Source: CAD feature listing. Evaluate the final solid. Frame: model axes, mm. A direction names the side the tool comes from. Give positions to 0.01 mm unless a question says otherwise; leave off trailing zeros. Order: outer loops, then holes, each group sorted by start corner. A loop starts at its lowest first (then second) coordinate and runs counter-clockwise, first axis right, second up. Notation, with made-up numbers: M 62.5,48.25 L 74.5,48.25 A6 ccw 74.5,59.25 Z; hole C 85.25,27 d10. An arc over 180 degrees is marked long. Answer in a Markdown table with one row per item. Add a question column.
(1) Section query C-C, the plane z = 2.8. Return loops of the section in (x, y) (3 decimals), plus the area to 3 significant figures.
(2) Section query D-D, the plane x = 14.5. Return loops of the section in (y, z), plus the area to 3 significant figures.
(3) Section query A-A, the plane x = 10.5. Return loops of the section in (y, z) (3 decimals), plus the area to 3 significant figures.
(4) Section query B-B, the plane z = 5.75. Return loops of the section in (x, y) (3 decimals).
(5) Mould query, pull axis Z, two halves, no side actions, for faces 1 (the face through (9.53, 33.74, 3.55)), 2 (the face through (21, 15, 6)), 3 (the face through (33.226, 12.769, 3.938)), 4 (the face through (20, 13, 0)). Classes: pulls with the +Z half, pulls with the -Z half, needs draft (parallel to the pull), parting line crosses it, or undercut.
(6) Material intervals for line 1 along X through (y, z) = (32.5, 2.75) (3 decimals); line 2 along Y through (x, z) = (19.75, 4.5); line 3 along Y through (x, z) = (14.5, 10.25), sorted ascending.
(7) Pin query (flat end, axial travel): P1, Ø12, axis at x = 26.5, y = 16.5, coming from the -Z side; P2, Ø1.5, axis at y = 28, z = 12, coming from the -X side; P3, Ø5, axis at x = 28, y = 25.5, coming from the -Z side; P4, Ø6, axis at y = 20, z = 12.5, coming from the +X side (3 decimals). Return the tip coordinate at first contact, or that it passes through.
(8) Set-up query: faces 5 (the face through (20, 23, 7.5)), 6 (the face through (10, 20, 11)), 7 (the face through (11.226, 12.769, 3.938)), 8 (the face through (21, 31, 6)), 9 (the face through (6.525, 13, 7)). Return all of +Z, -Z, +X, -X, +Y, -Y with unobstructed straight access to the full face (end or side cutting, diameter ignored); none if empty.
Autodesk Inventor part; units mm, degrees
ref_plane "YZ Plane" through (0, 0, 0) normal (1, 0, 0) x (0, 1, 0)
ref_plane "XZ Plane" through (0, 0, 0) normal (0, 1, 0) x (-1, 0, 0)
ref_plane "XY Plane" through (0, 0, 0) normal (0, 0, 1) x (1, 0, 0)
sketch "스케치1" plane through (0, 0, 0) normal (0, 0, 1) x (1, 0, 0)
  line L0 (7.5, 38) -> (7.5, 36.5)
  line L1 (2, 38) -> (7.5, 38)
  line L2 (2, 38) -> (2, 8)
  line L3 (2, 8) -> (6.525, 8)
  line L4 (6.525, 10.5) -> (6.525, 8)
  line L5 (6.525, 10.5) -> (10.3997, 10.5)
  line L6 (10.3997, 10.5) -> (10.6003, 10.5)
  line L7 (10.6003, 10.5) -> (14.475, 10.5)
  line L8 (14.475, 10.5) -> (14.475, 8)
  line L9 (14.475, 8) -> (28.525, 8)
  line L10 (28.525, 10.5) -> (28.525, 8)
  line L11 (28.525, 10.5) -> (32.3997, 10.5)
  line L12 (32.3997, 10.5) -> (32.6003, 10.5)
  line L13 (32.6003, 10.5) -> (34.7876, 10.5)
  line L14 (34.7876, 10.5) -> (34.7876, 19.4)
  line L15 (36, 19.4) -> (34.7876, 19.4)
  line L16 (36, 24) -> (36, 19.4)
  line L17 (38.55, 24) -> (36, 24)
  line L18 (38.55, 24) -> (38.55, 25.4)
  line L19 (38.55, 25.4) -> (37.1, 25.4)
  line L20 (37.1, 25.4) -> (37.1, 35.5)
  line L21 (49.9, 35.5) -> (37.1, 35.5)
  line L22 (49.9, 25.4) -> (49.9, 35.5)
  line L23 (49.9, 25.4) -> (48.45, 25.4)
  line L24 (48.45, 24) -> (48.45, 25.4)
  line L25 (51, 24) -> (48.45, 24)
  line L26 (51, 24) -> (51, 10.5)
  line L27 (51, 10.5) -> (54.3997, 10.5)
  line L28 (54.3997, 10.5) -> (54.6003, 10.5)
  line L29 (54.6003, 10.5) -> (57.5, 10.5)
  line L30 (57.5, 36.5) -> (57.5, 10.5)
  line L31 (57.5, 36.5) -> (51.5, 36.5)
  line L32 (51.5, 38) -> (51.5, 36.5)
  line L33 (35.5, 38) -> (51.5, 38)
  line L34 (35.5, 36.5) -> (35.5, 38)
  line L35 (35.5, 36.5) -> (29.5, 36.5)
  line L36 (29.5, 38) -> (29.5, 36.5)
  line L37 (13.5, 38) -> (29.5, 38)
  line L38 (13.5, 36.5) -> (13.5, 38)
  line L39 (13.5, 36.5) -> (7.5, 36.5)
  line L40 (22.05, 14.2) -> (27.95, 14.2)
  line L41 (22.05, 18) -> (22.05, 14.2)
  line L42 (27.95, 18) -> (22.05, 18)
  line L43 (27.95, 14.2) -> (27.95, 18)
  line L44 (34.6876, 10.6) -> (7.6, 10.6)
  line L45 (7.6, 10.6) -> (7.6, 36.4)
  line L46 (7.6, 36.4) -> (34.6876, 36.4)
  line L47 (34.6876, 36.4) -> (34.6876, 10.6)
  line L48 (7.6, 36.4) -> (6.525, 36.4)
  line L49 (7.6, 10.6) -> (6.525, 10.6)
  line L50 (6.525, 10.6) -> (6.525, 36.4)
  line L51 (6.525, 36.4) -> (7.6, 36.4)
  line L52 (7.6, 36.4) -> (7.6, 10.6)
  point P0 (0, 0)
extrude "돌출1" add sketch "스케치1" along normal blind 15 contours L41 L42 L43 L40 | L44 L45 L46 L47 | L49 L50 L48 L45
sketch "스케치2" plane through (0, 0, 15) normal (0, 0, 1) x (1, 0, 0)
  line L0 (34.5, 38) -> (52.5, 38)
  line L1 (52.5, 38) -> (52.5, 36.5)
  line L2 (56.5, 36.5) -> (52.5, 36.5)
  line L3 (56.5, 38) -> (56.5, 36.5)
  line L4 (56.5, 38) -> (59.1, 38)
  line L5 (59.1, 38) -> (59.1, 40)
  line L6 (6, 40) -> (59.1, 40)
  line L7 (6, 38) -> (6, 40)
  line L8 (6, 38) -> (8.5, 38)
  line L9 (8.5, 38) -> (8.5, 36.5)
  line L10 (12.5, 36.5) -> (8.5, 36.5)
  line L11 (12.5, 38) -> (12.5, 36.5)
  line L12 (12.5, 38) -> (30.5, 38)
  line L13 (30.5, 38) -> (30.5, 36.5)
  line L14 (34.5, 36.5) -> (30.5, 36.5)
  line L15 (34.5, 38) -> (34.5, 36.5)
  line L16 (14.475, 10.5) -> (12.975, 10.5)
  line L17 (12.975, 10.5) -> (12.975, 8.5)
  line L18 (12.975, 8.5) -> (8.025, 8.5)
  line L19 (8.025, 10.5) -> (8.025, 8.5)
  line L20 (8.025, 10.5) -> (6.525, 10.5)
  line L21 (6.525, 10.5) -> (6.525, 8)
  line L22 (6, 8) -> (6.525, 8)
  line L23 (6, 8) -> (6, 6)
  line L24 (6, 6) -> (59.1, 6)
  line L25 (59.1, 8) -> (59.1, 6)
  line L26 (58.475, 8) -> (59.1, 8)
  line L27 (58.475, 8) -> (58.475, 10.5)
  line L28 (58.475, 10.5) -> (56.975, 10.5)
  line L29 (56.975, 10.5) -> (56.975, 8.5)
  line L30 (56.975, 8.5) -> (52.025, 8.5)
  line L31 (52.025, 10.5) -> (52.025, 8.5)
  line L32 (52.025, 10.5) -> (50.525, 10.5)
  line L33 (50.525, 10.5) -> (50.525, 8)
  line L34 (36.475, 8) -> (50.525, 8)
  line L35 (36.475, 8) -> (36.475, 10.5)
  line L36 (36.475, 10.5) -> (34.975, 10.5)
  line L37 (34.975, 10.5) -> (34.975, 8.5)
  line L38 (34.975, 8.5) -> (30.025, 8.5)
  line L39 (30.025, 10.5) -> (30.025, 8.5)
  line L40 (30.025, 10.5) -> (28.525, 10.5)
  line L41 (28.525, 10.5) -> (28.525, 8)
  line L42 (14.475, 8) -> (28.525, 8)
  line L43 (14.475, 8) -> (14.475, 10.5)
  line L44 (14.475, 36.4) -> (28.525, 36.4)
  line L45 (34.6876, 10.6) -> (34.6876, 36.4)
  line L46 (14.475, 10.6) -> (28.525, 10.6)
  line L47 (28.525, 10.6) -> (28.525, 36.4)
  line L48 (28.525, 36.4) -> (14.475, 36.4)
  line L49 (-13.0231, 23) -> (78.1205, 23)
  line L50 (14.5, -11.1) -> (14.5, 56.1)
  line L51 (34.6876, 36.4) -> (6.525, 36.4)
  line L52 (6.525, 36.4) -> (6.525, 10.6)
  line L53 (6.525, 10.6) -> (34.6876, 10.6)
  line L54 (28.525, 23) -> (34.6876, 23)
  line L55 (34.6876, 23) -> (34.6876, 31)
  line L56 (34.6876, 31) -> (28.525, 31)
  line L57 (28.525, 31) -> (28.525, 23)
  line L58 (28.525, 23) -> (34.6876, 23)
  line L59 (34.6876, 23) -> (34.6876, 15)
  line L60 (34.6876, 15) -> (28.525, 15)
  line L61 (28.525, 15) -> (28.525, 23)
  line L62 (6.525, 23) -> (12.688, 23)
  line L63 (12.688, 23) -> (12.688, 31)
  line L64 (12.688, 31) -> (6.525, 31)
  line L65 (6.525, 31) -> (6.525, 23)
  line L66 (14.5, 57.1) -> (14.5, -10.1)
  line L67 (12.688, 23) -> (12.688, 15)
  line L68 (12.688, 15) -> (6.525, 15)
  line L69 (6.525, 15) -> (6.525, 23)
  line L70 (6.525, 36.4) -> (6.525, 10.6)
  line L71 (12.688, 23) -> (6.525, 23)
  line L72 (6.525, 23) -> (6.525, 26)
  line L73 (6.525, 26) -> (12.688, 26)
  line L74 (12.688, 26) -> (12.688, 23)
  line L75 (12.688, 23) -> (6.525, 23)
  line L76 (6.525, 23) -> (6.525, 20)
  line L77 (6.525, 20) -> (12.688, 20)
  line L78 (12.688, 20) -> (12.688, 23)
  point P0 (0, 0)
  dimension "d3" = 6.163
  dimension "d4" = 8
extrude "돌출2" cut sketch "스케치2" against normal up to next contours L56 L45 L49 L47 | L49 L45 L60 L47 | L64 L63 L73 L52 | L67 L68 L52 L77
sketch "스케치4" plane through (6.525, 10.6, 0) normal (0, -1, 0) x (1, 0, 0)
  circle A0 centre (3.975, 2.8) radius 1.35
  circle A1 centre (25.975, 2.8) radius 1.35
  circle A2 centre (25.975, 2.8) radius 1.55
  circle A3 centre (3.975, 2.8) radius 1.55
  point P0 (-6.525, 0)
  dimension "d14" = 0.2
  dimension "d15" = 0.2
extrude "돌출4" cut sketch "스케치4" against normal up to next contours A0 | A1
sketch "스케치5" plane through (6.525, 36.4, 0) normal (0, 1, 0) x (1, 0, 0)
  circle A0 centre (25.975, -2.8) radius 1.025
  circle A1 centre (3.975, -2.8) radius 1.025
  circle A2 centre (25.975, -2.8) radius 1.225
  circle A3 centre (3.975, -2.8) radius 1.225
  point P0 (-6.525, 0)
  dimension "d16" = 0.2
  dimension "d17" = 0.2
extrude "돌출5" cut sketch "스케치5" against normal up to next contours A0 | A1 | A2 | A3
sketch "스케치6" plane through (0, 0, 0) normal (0, 0, -1) x (-1, 0, 0)
  line L0 (-28.525, 31) -> (-34.6876, 31)
  line L1 (-34.6876, 31) -> (-34.6876, 36.4)
  line L2 (-34.6876, 36.4) -> (-6.525, 36.4)
  line L3 (-6.525, 36.4) -> (-6.525, 31)
  line L4 (-6.525, 31) -> (-12.688, 31)
  line L5 (-12.688, 31) -> (-12.688, 26)
  line L6 (-12.688, 26) -> (-6.525, 26)
  line L7 (-6.525, 26) -> (-6.525, 20)
  line L8 (-6.525, 20) -> (-12.688, 20)
  line L9 (-12.688, 20) -> (-12.688, 15)
  line L10 (-12.688, 15) -> (-6.525, 15)
  line L11 (-6.525, 15) -> (-6.525, 10.6)
  line L12 (-6.525, 10.6) -> (-34.6876, 10.6)
  line L13 (-34.6876, 10.6) -> (-34.6876, 15)
  line L14 (-34.6876, 15) -> (-28.525, 15)
  line L15 (-28.525, 15) -> (-28.525, 31)
  line L16 (-12.688, 31) -> (-28.525, 31)
  line L17 (-28.525, 31) -> (-28.525, 15)
  line L18 (-28.525, 15) -> (-12.688, 15)
  line L19 (-12.688, 15) -> (-12.688, 31)
  line L20 (13.0231, 24) -> (-78.1205, 24)
  line L21 (-14.5, 58.1) -> (-14.5, -9.1)
  point P0 (0, 0)
extrude "돌출6" cut sketch "스케치6" against normal blind 7.5 contours L16 L21 L20 L15 | L20 L21 L18 L15 | L16 L5 L19 L20 L21 | L20 L19 L9 L18 L21 | L20 L7 L8 L19 | L19 L6 L7 L20
sketch "스케치7" plane through (0, 0, 15) normal (0, 0, 1) x (1, 0, 0)
  circle A0 centre (14.5, 24) radius 1.55
  point P0 (0, 0)
extrude "돌출7" cut sketch "스케치7" against normal up to next
properties part number "foot_bridge"
Values follow:
| question | item | result |
|---|---|---|
| 1 | outline | M 6.525,10.6 L 9.15,10.6 L 9.15,15 L 6.525,15 Z; M 6.525,31 L 9.275,31 L 9.275,36.4 L 6.525,36.4 Z; M 11.725,31 L 31.275,31 L 31.275,36.4 L 11.725,36.4 Z; M 11.85,10.6 L 31.15,10.6 L 31.15,15 L 11.85,15 Z; M 33.725,31 L 34.688,31 L 34.688,36.4 L 33.725,36.4 Z; M 33.85,10.6 L 34.688,10.6 L 34.688,15 L 33.85,15 Z |
| 1 | area | 226 mm² |
| 2 | outline | M 10.6,0 L 15,0 L 15,7.5 L 22.45,7.5 L 22.45,15 L 10.6,15 Z; M 25.55,7.5 L 31,7.5 L 31,0 L 36.4,0 L 36.4,15 L 25.55,15 Z |
| 2 | area | 244 mm² |
| 3 | outline | M 10.6,0 L 15,0 L 15,1.45 L 10.6,1.45 Z; M 10.6,4.15 L 15,4.15 L 15,15 L 10.6,15 Z; M 20,7.5 L 26,7.5 L 26,15 L 20,15 Z; M 31,0 L 36.4,0 L 36.4,1.575 L 31,1.575 Z; M 31,4.025 L 36.4,4.025 L 36.4,15 L 31,15 Z |
| 3 | area | 167 mm² |
| 4 | outline | M 6.525,10.6 L 34.688,10.6 L 34.688,15 L 6.525,15 Z; M 6.525,31 L 34.688,31 L 34.688,36.4 L 6.525,36.4 Z |
| 5 | face 1 | undercut |
| 5 | face 2 | needs draft |
| 5 | face 3 | undercut |
| 5 | face 4 | pulls with the -Z half |
| 6 | line 1 | x = 6.525 to 9.276, 11.724 to 31.276, 33.724 to 34.688 |
| 6 | line 2 | y = 10.6 to 15, 31 to 36.4 |
| 6 | line 3 | y = 10.6 to 22.45, 25.55 to 36.4 |
| 7 | P1 | stops at z = 0 |
| 7 | P2 | stops at x = 12.69 |
| 7 | P3 | stops at z = 7.5 |
| 7 | P4 | stops at x = 28.525 |
| 8 | face 5 | -Z, +X, -X |
| 8 | face 6 | +Z, -Z, -X |
| 8 | face 7 | -Y |
| 8 | face 8 | -Z |
| 8 | face 9 | +Z, -Z, -X, +Y, -Y |
